Geometry: see drawing. Coordinates: mm, zero at the bounding-box minimum. Coordinates: 2 decimals unless noted, no trailing zeros. Order: outer loops, then holes, each group sorted by start corner. A loop starts at its lowest first (then second) coordinate and runs counter-clockwise, first axis right, second up. Notation, with made-up numbers: (77, 39) - (115, 39) arc R33 cw to (115, 69) - close; hole circle Ø6 at (27.25, 57.25). An arc over 180 degrees is marked (long way). Use a Markdown table: item, result. Add a question column.
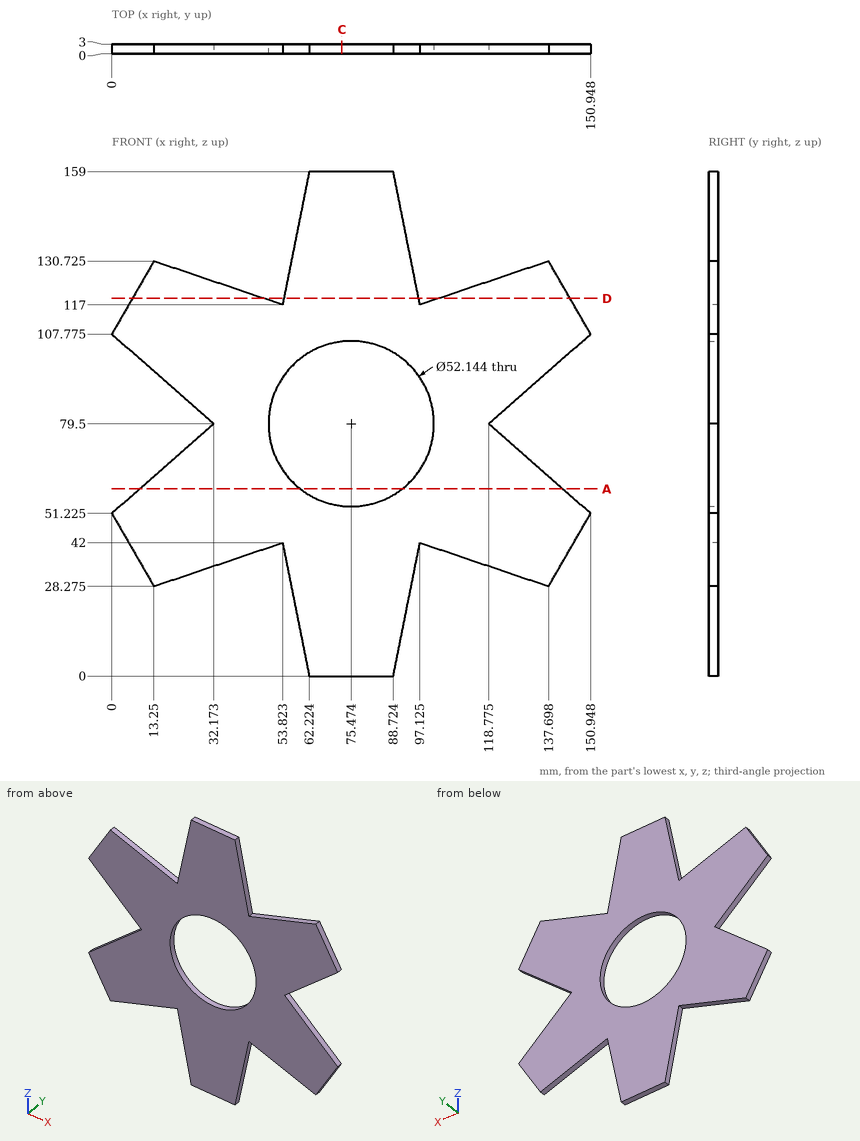
1) First-contact query: pin 1 (1 mm diameter, centred on y = 1, z = 110.5, fed in from +X); pin 2 (1 mm diameter, centred on x = 109, y = 0.5, fed in from +Z); pin 3 (1 mm diameter, centred on y = 2.5, z = 108.5, fed in from -X); pin 4 (4 mm diameter, centred on x = 52, z = 56, fed in from -Y). Flat tips, straight axial feed; report the tip coordinate or a pass-through.
2) Line query: line 1 (Z direction, x = 74, y = 1); line 2 (Z direction, x = 84, y = 1.45); line 3 (Z direction, x = 39, y = 0.6) (1 decimal). Output: solid intervals per line, ascending. Write a range as from..to.
3) Section query D-D (z = 119). Return the cut outline in (x, y) (1 decimal), and give its area (3 significant figures).
4) Section query C-C (x = 72.5). Return the cut outline in (y, z).
5) Section query A-A (z = 59). Return the cut outline in (x, y) (1 decimal).
From the geometry:
| question | item | result |
|---|---|---|
| 1 | pin 1 | stops at x = 149.66 |
| 1 | pin 2 | stops at z = 121.19 |
| 1 | pin 3 | stops at x = 0.13 |
| 1 | pin 4 | stops at y = 0 |
| 2 | line 1 | z = 0..53.47, 105.53..159 |
| 2 | line 2 | z = 0..54.86, 104.14..159 |
| 2 | line 3 | z = 37..122 |
| 3 | outline | (6.5, 0) - (47.9, 0) - (47.9, 3) - (6.5, 3) - close; (54.2, 0) - (96.7, 0) - (96.7, 3) - (54.2, 3) - close; (103, 0) - (144.5, 0) - (144.5, 3) - (103, 3) - close |
| 3 | area | 376 mm^2 |
| 4 | outline | (0, 0) - (3, 0) - (3, 53.6) - (0, 53.6) - close; (0, 105.4) - (3, 105.4) - (3, 159) - (0, 159) - close |
| 5 | outline | (8.8, 0) - (59.4, 0) - (59.4, 3) - (8.8, 3) - close; (91.6, 0) - (142.1, 0) - (142.1, 3) - (91.6, 3) - close |
